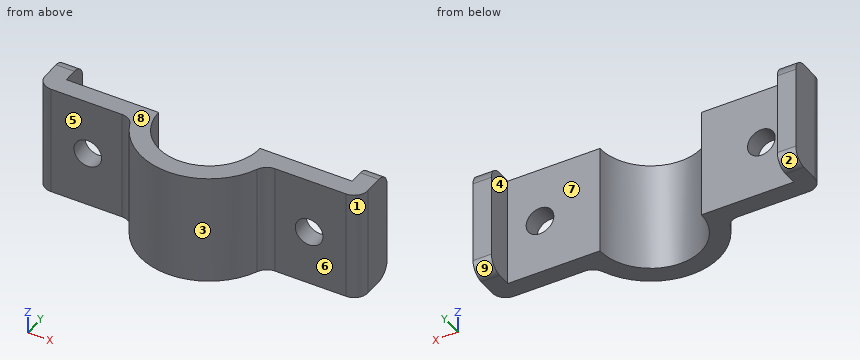
from build123d import *

# Parameters (mm, degrees)
F1_DEPTH = 76.2
F2_R     = 9.525
F3_DEPTH = 31.751
F4_R     = 9.525


with BuildPart() as f1:
    # F0 (on Top) → F1 (new body)
    with BuildSketch(Plane.XY):
        with BuildLine():
            Line((-98.425, 19.05), (-111.125, 19.05))
            Line((-111.125, 19.05), (-111.125, -12.7))
            Line((-111.125, -12.7), (-45.900443, -12.7))
            ThreePointArc((-45.900443, -12.7), (0, -47.625), (45.900443, -12.7))
            Line((45.900443, -12.7), (111.125, -12.7))
            Line((111.125, -12.7), (111.125, 19.05))
            Line((111.125, 19.05), (98.425, 19.05))
            Line((98.425, 19.05), (98.425, 0))
            Line((98.425, 0), (34.925, 0))
            ThreePointArc((34.925, 0), (0, -34.925), (-34.925, 0))
            Line((-34.925, 0), (-98.425, 0))
            Line((-98.425, 0), (-98.425, 19.05))
        make_face()
    extrude(amount=F1_DEPTH)

    # F2 (on face) → F3 (cut, through all)
    with BuildSketch(Plane.XZ.offset(12.7)):
        with Locations((-76.2, 38.1)):
            Circle(F2_R)
        with Locations((76.2, 38.1)):
            Circle(F2_R)
    extrude(amount=-F3_DEPTH, mode=Mode.SUBTRACT)

    # F4
    f4_edges = [f1.edges().sort_by_distance(p)[0] for p in [
        (111.125, -12.7, 38.1),
        (45.900443, -12.7, 38.1),
        (-45.900443, -12.7, 38.1),
        (-111.125, -12.7, 38.1),
        (104.775, 19.05, 76.2),
        (-104.775, 19.05, 76.2),
        (104.775, 19.05, 0),
        (-104.775, 19.05, 0),
    ]]
    fillet(f4_edges, radius=F4_R)


solid = f1.part
CAD build for the part. Positions are in the model's coordinates, mm. Face numbers are marked on the shaded views. A direction names the side the tool comes from. Round coordinates to 2 decimals unless told otherwise and drop trailing zeros. Write each loop counter-clockwise with the first axis right and the second up, starting at its lowest first coordinate (ties: lowest second). Pieces come first, ordered by that corner, then holes.
(1) Mould opens along X. For the marked faces 1, 2, 3 and 4 say: pulls with the +X half, pulls with the -X half, needs draft (parallel to the pull), parting line crosses it, or undercut.
(2) Drop flat-ended pins along their axis: P1, Ø5, axis at x = 4.5, y = -30, coming from the -Z side; P2, Ø12, axis at x = -31, z = 27.5, coming from the +Y side; P3, Ø3, axis at y = -10, z = 21.5, coming from the -X side; P4, Ø24.5, axis at x = 74.5, z = 45, coming from the -Y side. Give the stop position or say it passes through.
(3) Slice it at C-C, the plane y = -9. Write the cut outline in (x, z) (3 decimals), and give its area (3 significant figures).
(4) Slice it at D-D, the plane y = -22. Write the cut outline in (x, z), and give its area (3 significant figures).
(5) Probe line 1 along Z through (x, y) = (77, -8.5); line 2 along X through (y, z) = (11.5, 21.5) (3 decimals); line 3 along X through (y, z) = (-1, 55) (3 decimals). List the from-to ranges inside material, lowest first.
(6) Slice it at A-A, the plane x = 76.2. Write the cut outline in (y, z) (3 decimals), and give its area (3 significant figures).
(7) 3-axis set-ups, long thin cutter, end or side, ignore diameter. For the marked faces 5, 6, 7, 8 and 9: which of +Z, -Z, +X, -X, +Y, -Y reach the whole face in a straight line?
(8) Slice it at B-B, the plane z = 38.1. Write the cut outline in (x, y) (3 decimals).
From the geometry:
1. face 1: pulls with the +X half
1. face 2: needs draft
1. face 3: parting line crosses it
1. face 4: undercut
2. P1: passes through
2. P2: stops at y = 0
2. P3: stops at x = -109.5
2. P4: stops at y = -12.7
3. outline: (-109.136, 0) - (-33.745, 0) - (-33.745, 76.2) - (-109.136, 76.2) - close; (33.745, 0) - (109.136, 0) - (109.136, 76.2) - (33.745, 76.2) - close; hole circle Ø19.05 at (-76.2, 38.1); hole circle Ø19.05 at (76.2, 38.1)
3. area: 10,900 mm2
4. outline: (-42.24, 0) - (-27.12, 0) - (-27.12, 76.2) - (-42.24, 76.2) - close; (27.12, 0) - (42.24, 0) - (42.24, 76.2) - (27.12, 76.2) - close
4. area: 2,300 mm2
5. line 1: z = 0 to 28.61, 47.59 to 76.2
5. line 2: x = -111.125 to -98.425, 98.425 to 111.125
5. line 3: x = -111.125 to -34.911, 34.911 to 111.125
6. outline: (-12.7, 0) - (0, 0) - (0, 28.575) - (-12.7, 28.575) - close; (-12.7, 47.625) - (0, 47.625) - (0, 76.2) - (-12.7, 76.2) - close
6. area: 726 mm2
7. face 5: +Z, -Z, -X, -Y
7. face 6: +Z, -Z, +X, -Y
7. face 7: +Z, -Z, +Y
7. face 8: +Z, +X, -X, +Y, -Y
7. face 9: -Z, +X, -X, +Y
8. outline: (-111.125, -3.175) arc R9.525 ccw to (-101.6, -12.7) - (-85.725, -12.7) - (-85.725, 0) - (-98.425, 0) - (-98.425, 19.05) - (-111.125, 19.05) - close; (-66.675, -12.7) - (-52.651, -12.7) arc R9.525 cw to (-43.876, -18.521) arc R47.625 ccw to (43.876, -18.521) arc R9.525 cw to (52.651, -12.7) - (66.675, -12.7) - (66.675, 0) - (34.925, 0) arc R34.925 cw to (-34.925, 0) - (-66.675, 0) - close; (85.725, -12.7) - (101.6, -12.7) arc R9.525 ccw to (111.125, -3.175) - (111.125, 19.05) - (98.425, 19.05) - (98.425, 0) - (85.725, 0) - close
